The figure shows three views and two pictorial views of one solid part (mm, origin at its lowest corner). Answer the questions. A direction names the side the tool comes from. Coordinates: 2 decimals unless noted, no trailing zeros. Write each loop counter-clockwise with the first axis right and the second up, starting at its lowest first coordinate (ties: lowest second). Pieces come first, ordered by that corner, then holes.
Item 1: Straight lines are drawn through the part: probe 1 along Y at (x, z) = (25, 6.75); probe 2 along Z at (x, y) = (25, 42.75); probe 3 along Z at (x, y) = (32.5, 6). For each, find the intervals that lie inside material, in ascending order.
Item 2: Section A-A (x = 31) is taken. Give the vertices of the cut face in (y, z), then the cut area to 3 significant figures.
Item 3: Section C-C (x = 25) is taken. Give the vertices of the cut face in (y, z), then the cut area to 3 significant figures.
Item 4: Determine the mould class of the marked faces 3, 4, 5 and 6 for opening direction X: released by +X, released by -X, zero draft, split by the parting line, or undercut.
Item 5: A tool of negligible diameter and unlimited length cuts with its end or side. For the marked faces 1 and 2, from which of +Z, -Z, +X, -X, +Y, -Y can it reach the whole face along a straight path? Write none if from no direction.
Item 6: Section B-B (y = 25) is taken. Give the vertices of the cut face in (x, z).
Item 7: Section D-D (z = 60) is taken. Give the vertices of the cut face in (x, y), then the cut area to 3 significant figures.
Item 8: Each of these flat-tipped pins is pushed along its axis until it touches: P1, Ø6, axis at x = 30.5, y = 43.5, coming from the -Z side; P2, Ø4, axis at x = 35, z = 29.5, coming from the -Y side; P3, Ø23, axis at x = 25, y = 25, coming from the +Z side. Where does it stop, or does it pass through?
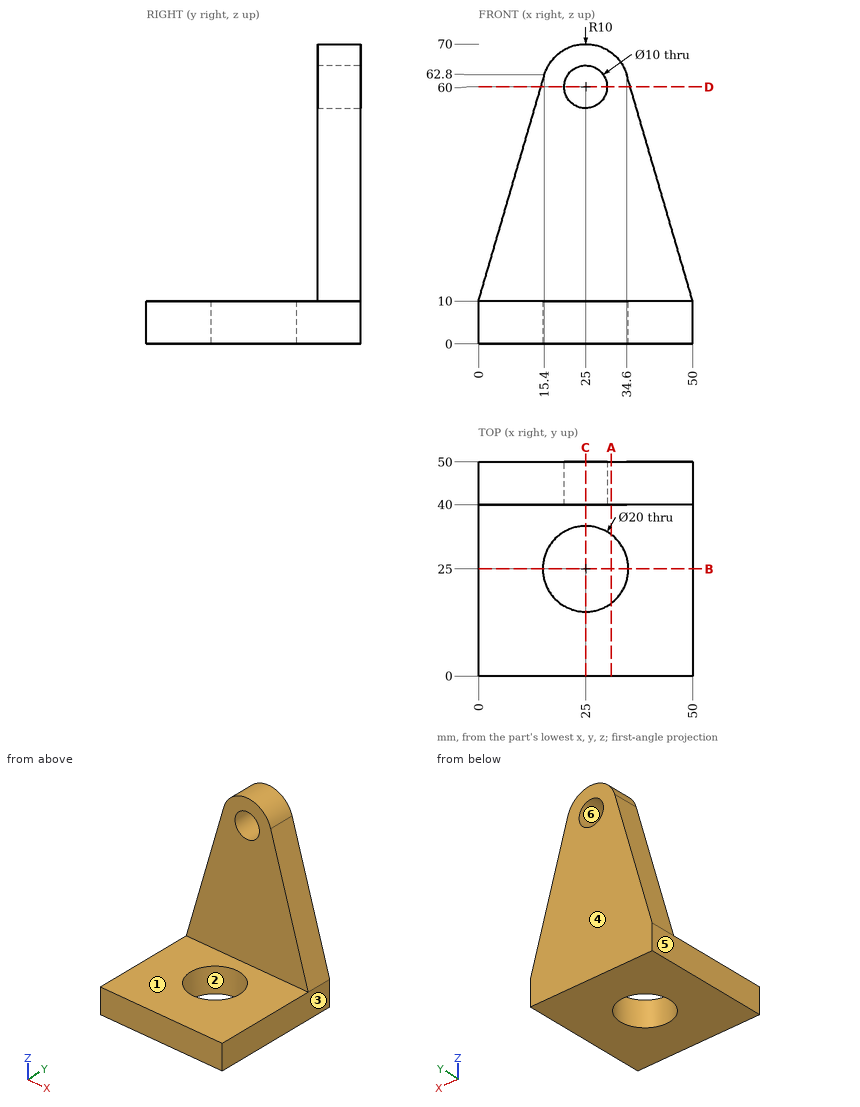
Established:
1. probe 1: y = 0 to 15, 35 to 50
1. probe 2: z = 0 to 55, 65 to 70
1. probe 3: z = 0 to 10
2. outline: (0, 0) - (17, 0) - (17, 10) - (0, 10) - close; (33, 0) - (50, 0) - (50, 68) - (40, 68) - (40, 10) - (33, 10) - close
2. area: 920 mm2
3. outline: (0, 0) - (15, 0) - (15, 10) - (0, 10) - close; (35, 0) - (50, 0) - (50, 55) - (40, 55) - (40, 10) - (35, 10) - close; (40, 65) - (50, 65) - (50, 70) - (40, 70) - close
3. area: 800 mm2
4. face 3: released by +X
4. face 4: zero draft
4. face 5: released by -X
4. face 6: undercut
5. face 1: +Z, +X, -X, -Y
5. face 2: +Z, -Z
6. outline: (0, 0) - (15, 0) - (15, 10) - (0, 10) - close; (35, 0) - (50, 0) - (50, 10) - (35, 10) - close
7. outline: (14.58, 40) - (20, 40) - (20, 50) - (14.58, 50) - close; (30, 40) - (35.42, 40) - (35.42, 50) - (30, 50) - close
7. area: 108 mm2
8. P1: stops at z = 0
8. P2: stops at y = 40
8. P3: stops at z = 10
